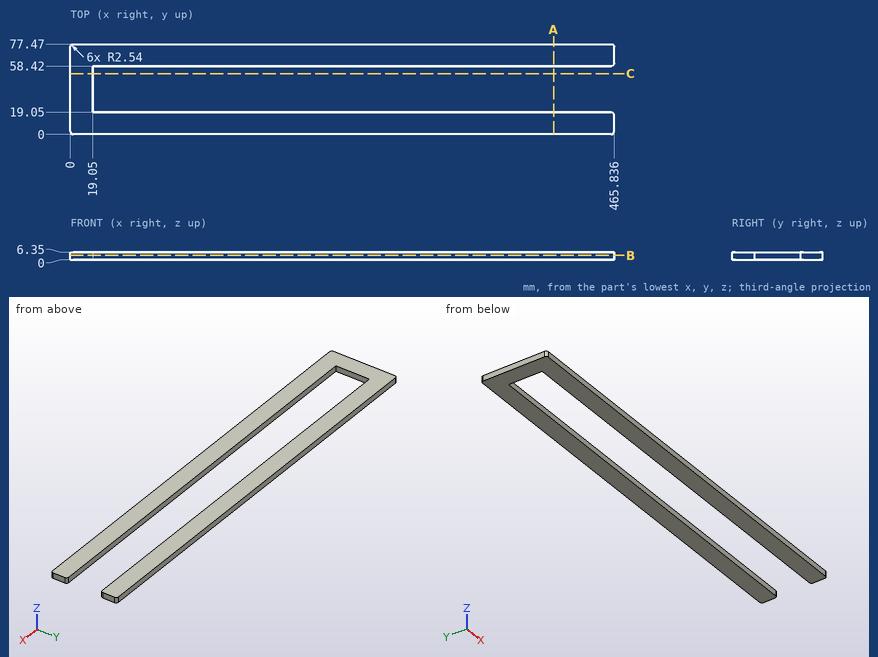
Drawing for the job (mm, zero at the part's lowest x, y, z). Give positions to 0.01 mm unless a question says otherwise; leave off trailing zeros. Loops run counter-clockwise (first coordinate to the right, second up) from the corner with the lowest first, then second, coordinate; pieces in that order, holes last.
(1) Pin check, flat tips, straight feed: pin 1 (4 mm diameter, centred on x = 383, y = 12, fed in from -Z); pin 2 (8 mm diameter, centred on x = 296, y = 25.5, fed in from -Z). Stop position of each tip, or through.
Return value:
pin 1: stops at z = 0
pin 2: passes through
(2) Band-saw the part on A-A (x = 414). Write the cut outline in (y, z).
Return value:
outline: (0, 0) - (19.05, 0) - (19.05, 6.35) - (0, 6.35) - close; (58.42, 0) - (77.47, 0) - (77.47, 6.35) - (58.42, 6.35) - close
(3) Drill centre lines: line 1 along Y through (x, z) = (439, 1.75); line 2 along X through (y, z) = (45, 4.25). Where is each one in solid material? Low to high.
Return value:
line 1: y = 0 to 19.05, 58.42 to 77.47
line 2: x = 0 to 19.05
(4) Band-saw the part on C-C (y = 52). Write the cut outline in (x, z), and give its area (3 significant figures).
Return value:
outline: (0, 0) - (19.05, 0) - (19.05, 6.35) - (0, 6.35) - close
area: 121 mm2
(5) Band-saw the part on B-B (z = 3.75). Write the cut outline in (x, y).
Return value:
outline: (0, 2.54) arc R2.54 ccw to (2.54, 0) - (463.3, 0) arc R2.54 ccw to (465.84, 2.54) - (465.84, 16.51) arc R2.54 ccw to (463.3, 19.05) - (19.05, 19.05) - (19.05, 58.42) - (463.3, 58.42) arc R2.54 ccw to (465.84, 60.96) - (465.84, 74.93) arc R2.54 ccw to (463.3, 77.47) - (2.54, 77.47) arc R2.54 ccw to (0, 74.93) - close
